Here's how the part is built. I have some questions about the finished solid (model axes, mm). A direction names the side the tool comes from. Coordinates: 2 decimals unless noted, no trailing zeros. Write each loop counter-clockwise with the first axis right and the second up, starting at its lowest first coordinate (ties: lowest second). Pieces come first, ordered by that corner, then holes.
Item 1: I'm going to push a flat-ended pin straight in: pin 1 Ø3.5 at (x, z) = (0, 10.86) entering from +Y. Where does the tip first touch, or does it pass through?
Item 2: For faces 4 (the face through (0.282, 1.671, 9.588)), 5 (the face through (0, 0, 5)), 6 (the face through (0, 8.65, 2)), 7 (the face through (0, -2.95, 6)), 8 (the face through (0, 3.15, 9)), which set-ups out of +Z, -Z, +X, -X, +Y, -Y let a thin tool reach every point of the face, with its end or its side?
Item 3: If we section it at D-D (y = 1): Please give me the cut outline in (x, z), then the cut area to 3 significant figures.
Item 4: We'd pull the mould along X, two halves only. Please class faces 1 (the face through (0, 0.15, 9)), 2 (the face through (-3, 2, 5)), 3 (the face through (0.282, 1.671, 5.588)): +X half, -X half, draft (parallel to the pull), parting line (faces both ways), or undercut.
Item 5: If I drill on line 1 (Z direction, x = 0, y = 1.35); line 2 (X direction, y = 6, z = 1); line 3 (Z direction, x = 0.75, y = 0.25), over which ranges is the centre line in solid material (lowest first)?
Item 6: If we section it at B-B (z = 3.25): Please give me the cut outline in (x, y), then the cut area to 3 significant figures.
Item 7: If we section it at A-A (y = 5.9): Please give me the cut outline in (x, z).
Item 8: If we section it at C-C (x = 0): Count the separate pieces of the cut face and the enclosed holes in it, then the cut area to 3 significant figures.
from build123d import *

# Parameters (mm, degrees)
BOSS_EXTRUDE1_DEPTH     = 13
SKETCH6_W               = 6
SKETCH6_H               = 5
BOSS_EXTRUDE4_DEPTH     = 5.6
SKETCH16_W              = 6
SKETCH16_H              = 8
BOSS_EXTRUDE5_DEPTH     = 0.1
CUT_EXTRUDE6_DEPTH      = 4
CUT_EXTRUDE6_DEPTH_BACK = 3.6
SKETCH15_R              = 1.3
CUT_EXTRUDE7_DEPTH      = 8.7202
CUT_EXTRUDE8_START      = -0.2202
SKETCH19_W              = 6
SKETCH19_H              = 8
SKETCH19_R              = 1.3
CUT_EXTRUDE8_DEPTH      = 0.2202
SKETCH12_R              = 1.5
CUT_EXTRUDE5_DEPTH      = 6
CHAMFER1_SIZE           = 0.2
SKETCH20_W              = 5
SKETCH20_H              = 5.5
BOSS_EXTRUDE6_DEPTH     = 0.5
SKETCH21_W              = 5
SKETCH21_H              = 5.5
BOSS_EXTRUDE7_DEPTH     = 0.5
CHAMFER2_SIZE           = 0.2
CROQUIS1_W              = 5
CROQUIS1_H              = 5.5
CORTAR_EXTRUIR1_DEPTH   = 0.5
CROQUIS2_W              = 5
CROQUIS2_H              = 5.5
CORTAR_EXTRUIR2_DEPTH   = 1


with BuildPart() as part:
    # Sketch1 → Boss-Extrude1 (new body)
    with BuildSketch(Plane.XY):
        Polygon((3, 3.05), (3, -2.253801214), (2.388188946, -2.95), (-2.388188946, -2.95), (-3, -2.253801214), (-3, 3.05), align=None)
    extrude(amount=BOSS_EXTRUDE1_DEPTH)

    # Sketch6 → Boss-Extrude4 (add)
    with BuildSketch(Plane(origin=(0, 3.05, 0), x_dir=(1, 0, 0), z_dir=(0, 1, 0))):
        with Locations((0, -2.5)):
            Rectangle(SKETCH6_W, SKETCH6_H)
    extrude(amount=BOSS_EXTRUDE4_DEPTH)

    # Sketch16 → Boss-Extrude5 (add)
    with BuildSketch(Plane(origin=(0, 3.05, 0), x_dir=(1, 0, 0), z_dir=(0, 1, 0))):
        with Locations((0, -9)):
            Rectangle(SKETCH16_W, SKETCH16_H)
    extrude(amount=BOSS_EXTRUDE5_DEPTH)

    # Sketch18 → Cut-Extrude6 (cut, two sides: drawn at the far end of the back side and taken through both)
    with BuildSketch(Plane(origin=(0, 0, 0), x_dir=(0, 0, -1), z_dir=(1, 0, 0)).offset(-CUT_EXTRUDE6_DEPTH_BACK)):
        with BuildLine():
            Line((-8.8572, -0.0702), (-12.8572, -0.0702))
            Line((-12.8572, -0.0702), (-13, -0.0702))
            Line((-13, -0.0702), (-13, -0.7))
            Line((-13, -0.7), (-12.8572, -0.7))
            Line((-12.8572, -0.7), (-12.7144, -0.7))
            add(Edge.make_bspline(
                [(-12.7144, -0.7), (-12.5198, -0.7), (-12.43, -0.9509)],
                knots=[0.103448276, 0.103448276, 0.103448276, 0.137931034, 0.137931034, 0.137931034], degree=2))
            add(Edge.make_bspline(
                [(-12.43, -0.9509), (-12.3594, -1.2388), (-12.13, -1.45), (-11.8572, -1.45)],
                knots=[0.137931034, 0.137931034, 0.137931034, 0.137931034, 0.172413793, 0.172413793, 0.172413793, 0.172413793], degree=3))
            add(Edge.make_bspline(
                [(-11.8572, -1.45), (-11.5844, -1.45), (-11.355, -1.2388), (-11.2844, -0.9509)],
                knots=[0.172413793, 0.172413793, 0.172413793, 0.172413793, 0.206896552, 0.206896552, 0.206896552, 0.206896552], degree=3))
            add(Edge.make_bspline(
                [(-11.2844, -0.9509), (-11.1946, -0.7), (-11, -0.7)],
                knots=[0.206896552, 0.206896552, 0.206896552, 0.24137931, 0.24137931, 0.24137931], degree=2))
            Line((-11, -0.7), (-10.8572, -0.7))
            Line((-10.8572, -0.7), (-10.7144, -0.7))
            add(Edge.make_bspline(
                [(-10.7144, -0.7), (-10.5198, -0.7), (-10.43, -0.9509)],
                knots=[0.310344828, 0.310344828, 0.310344828, 0.344827586, 0.344827586, 0.344827586], degree=2))
            add(Edge.make_bspline(
                [(-10.43, -0.9509), (-10.3594, -1.2388), (-10.13, -1.45), (-9.8572, -1.45)],
                knots=[0.344827586, 0.344827586, 0.344827586, 0.344827586, 0.379310345, 0.379310345, 0.379310345, 0.379310345], degree=3))
            add(Edge.make_bspline(
                [(-9.8572, -1.45), (-9.5844, -1.45), (-9.355, -1.2388), (-9.2844, -0.9509)],
                knots=[0.379310345, 0.379310345, 0.379310345, 0.379310345, 0.413793103, 0.413793103, 0.413793103, 0.413793103], degree=3))
            add(Edge.make_bspline(
                [(-9.2844, -0.9509), (-9.1946, -0.7), (-9, -0.7)],
                knots=[0.413793103, 0.413793103, 0.413793103, 0.448275862, 0.448275862, 0.448275862], degree=2))
            Line((-9, -0.7), (-8.8572, -0.7))
            Line((-8.8572, -0.7), (-8.7144, -0.7))
            add(Edge.make_bspline(
                [(-8.7144, -0.7), (-8.5198, -0.7), (-8.43, -0.9509)],
                knots=[0.517241379, 0.517241379, 0.517241379, 0.551724138, 0.551724138, 0.551724138], degree=2))
            add(Edge.make_bspline(
                [(-8.43, -0.9509), (-8.3594, -1.2388), (-8.13, -1.45), (-7.8572, -1.45)],
                knots=[0.551724138, 0.551724138, 0.551724138, 0.551724138, 0.586206897, 0.586206897, 0.586206897, 0.586206897], degree=3))
            add(Edge.make_bspline(
                [(-7.8572, -1.45), (-7.5844, -1.45), (-7.355, -1.2388), (-7.2844, -0.9509)],
                knots=[0.586206897, 0.586206897, 0.586206897, 0.586206897, 0.620689655, 0.620689655, 0.620689655, 0.620689655], degree=3))
            add(Edge.make_bspline(
                [(-7.2844, -0.9509), (-7.1946, -0.7), (-7, -0.7)],
                knots=[0.620689655, 0.620689655, 0.620689655, 0.655172414, 0.655172414, 0.655172414], degree=2))
            Line((-7, -0.7), (-6.8572, -0.7))
            Line((-6.8572, -0.7), (-6.7144, -0.7))
            add(Edge.make_bspline(
                [(-6.7144, -0.7), (-6.5198, -0.7), (-6.43, -0.9509)],
                knots=[0.724137931, 0.724137931, 0.724137931, 0.75862069, 0.75862069, 0.75862069], degree=2))
            add(Edge.make_bspline(
                [(-6.43, -0.9509), (-6.3594, -1.2388), (-6.13, -1.45), (-5.8572, -1.45)],
                knots=[0.75862069, 0.75862069, 0.75862069, 0.75862069, 0.793103448, 0.793103448, 0.793103448, 0.793103448], degree=3))
            add(Edge.make_bspline(
                [(-5.8572, -1.45), (-5.5844, -1.45), (-5.355, -1.2388), (-5.2844, -0.9509)],
                knots=[0.793103448, 0.793103448, 0.793103448, 0.793103448, 0.827586207, 0.827586207, 0.827586207, 0.827586207], degree=3))
            add(Edge.make_bspline(
                [(-5.2844, -0.9509), (-5.1946, -0.7), (-5, -0.7)],
                knots=[0.827586207, 0.827586207, 0.827586207, 0.862068966, 0.862068966, 0.862068966], degree=2))
            Line((-5, -0.7), (-5, -0.0702))
            Line((-5, -0.0702), (-8.8572, -0.0702))
        make_face()
    extrude(amount=CUT_EXTRUDE6_DEPTH + CUT_EXTRUDE6_DEPTH_BACK, mode=Mode.SUBTRACT)

    # Sketch15 → Cut-Extrude7 (cut)
    with BuildSketch(Plane(origin=(0, 8.65, 0), x_dir=(1, 0, 0), z_dir=(0, 1, 0))):
        with Locations(Location((0, -10.8572, 0), (0, 0, 180))):
            Circle(SKETCH15_R)
        with Locations(Location((0, -6.8572, 0), (0, 0, 180))):
            Circle(SKETCH15_R)
    extrude(amount=-CUT_EXTRUDE7_DEPTH, mode=Mode.SUBTRACT)

    # Sketch19 → Cut-Extrude8 (cut)
    with BuildSketch(Plane.XZ.offset(0.0702).offset(CUT_EXTRUDE8_START)):
        with Locations((0, 9)):
            Rectangle(SKETCH19_W, SKETCH19_H)
        with Locations(Location((0, 10.8572, 0), (0, 0, 180))):
            Circle(SKETCH19_R, mode=Mode.SUBTRACT)
        with Locations(Location((0, 6.8572, 0), (0, 0, 180))):
            Circle(SKETCH19_R, mode=Mode.SUBTRACT)
    extrude(amount=CUT_EXTRUDE8_DEPTH, mode=Mode.SUBTRACT)

    # Sketch12 → Cut-Extrude5 (cut)
    with BuildSketch(Plane.XY.offset(5)):
        with Locations((0, 5.9)):
            Circle(SKETCH12_R)
    extrude(amount=-CUT_EXTRUDE5_DEPTH, mode=Mode.SUBTRACT)

    # Chamfer1
    chamfer1_edges = [part.edges().sort_by_distance(p)[0] for p in [
        (-2.694094473, -2.601900607, 13),
        (0, -2.95, 13),
        (2.694094473, -2.601900607, 13),
        (3, 1.65, 13),
        (3, -1.476900607, 13),
        (-3, -1.476900607, 13),
        (-3, 1.65, 13),
    ]]
    chamfer(chamfer1_edges, length=CHAMFER1_SIZE)

    # Sketch20 → Boss-Extrude6 (add)
    with BuildSketch(Plane(origin=(3, 0, 0), x_dir=(0, 0, -1), z_dir=(1, 0, 0))):
        with Locations((-2.5, 5.9)):
            Rectangle(SKETCH20_W, SKETCH20_H)
    extrude(amount=BOSS_EXTRUDE6_DEPTH)

    # Sketch21 → Boss-Extrude7 (add)
    with BuildSketch(Plane.ZY.offset(3)):
        with Locations((2.5, 5.9)):
            Rectangle(SKETCH21_W, SKETCH21_H)
    extrude(amount=BOSS_EXTRUDE7_DEPTH)

    # Chamfer2
    chamfer2_edges = [part.edges().sort_by_distance(p)[0] for p in [
        (3.5, 5.9, 5),
        (-3.5, 5.9, 5),
    ]]
    chamfer(chamfer2_edges, length=CHAMFER2_SIZE)

    # Croquis1 → Cortar-Extruir1 (cut)
    with BuildSketch(Plane.ZY.offset(3.5)):
        with Locations((2.5, 5.9)):
            Rectangle(CROQUIS1_W, CROQUIS1_H)
    extrude(amount=-CORTAR_EXTRUIR1_DEPTH, mode=Mode.SUBTRACT)

    # Croquis2 → Cortar-Extruir2 (cut)
    with BuildSketch(Plane(origin=(3, 0, 0), x_dir=(0, 0, -1), z_dir=(1, 0, 0))):
        with Locations((-2.5, 5.9)):
            Rectangle(CROQUIS2_W, CROQUIS2_H)
    extrude(amount=CORTAR_EXTRUIR2_DEPTH, mode=Mode.SUBTRACT)


solid = part.part
Answer list:
1. pin 1: stops at y = 3.15
2. face 4: +Y
2. face 5: +Z, +X, -X
2. face 6: +Z, -Z, +X, -X, +Y
2. face 7: +Z, -Z, +X, -X, -Y
2. face 8: +Z, +X, -X, +Y
3. outline: (-3, 0) - (3, 0) - (3, 12.8) - (2.8, 13) - (-2.8, 13) - (-3, 12.8) - close; hole circle Ø2.6 at (0, 6.86); hole circle Ø2.6 at (0, 10.86)
3. area: 67.3 mm2
4. face 1: draft
4. face 2: -X half
4. face 3: undercut
5. line 1: z = 0 to 5.56, 8.16 to 9.56, 12.16 to 13
5. line 2: x = -3 to -1.5, 1.5 to 3
5. line 3: z = 0 to 5.8, 7.92 to 9.8, 11.92 to 13
6. outline: (-3, -2.25) - (-2.39, -2.95) - (2.39, -2.95) - (3, -2.25) - (3, 8.65) - (-3, 8.65) - close; hole circle Ø3 at (0, 5.9)
6. area: 62.1 mm2
7. outline: (-3, 0) - (-1.5, 0) - (-1.5, 5) - (-3, 5) - close; (1.5, 0) - (3, 0) - (3, 5) - (1.5, 5) - close
8. separate pieces: 4
8. enclosed holes: 0
8. area: 66.4 mm2
